Can you work these out from the model? Positions are in its coordinate system, mm. A direction names the side the tool comes from. Round coordinates to 2 decimals unless told otherwise and drop trailing zeros. Order: outer loops, then holes, each group sorted by start corner. A loop starts at its lowest first (then second) coordinate and runs counter-clockwise, first axis right, second up.
Q1. If we section it at C-C (z = 332): Please give me the cut outline in (x, y), plus the area to 3 significant figures.
Q2. We'd pull the mould along Z, two halves only. Please class faces 4 (the face through (-856, 0, -168)), 5 (the face through (-5, 6.35, 2)), 6 (the face through (819, 6.35, 2)), 7 (the face through (-17, 163, -190.5)): pulls with the +Z half, pulls with the -Z half, needs draft (parallel to the pull), parting line crosses it, or undercut.
Q3. If we section it at B-B (z = -5): Please give me the cut outline in (x, y), plus the area to 3 significant figures.
Q4. For faces 1 (the face through (-829, 6.35, 2)), 2 (the face through (-100.41, 240.65, 280.64)), 3 (the face through (-1233.488, 163, -3)), which set-ups out of +Z, -Z, +X, -X, +Y, -Y let a thin tool reach every point of the face, with its end or its side?
Q5. If I drill on line 1 (Y direction, x = -34, z = -142); line 2 (Z direction, x = -452.5, y = 53.5); line 3 (Y direction, x = -56.5, z = 498.5), over which ranges is the centre line in solid material (lowest first)?
Q6. Will these pins go through, and if not, where does the flat tip stop? P1, Ø12, axis at x = 708, y = 263.5, coming from the +Z side; P2, Ø8, axis at x = -379, z = -47.5, coming from the +Y side.
Q7. If we section it at A-A (x = 56.5): Please give me the cut outline in (y, z), plus the area to 3 significant figures.
from build123d import *

# Parameters (mm, degrees)
F0_W     = 2466.975
F0_H     = 381
F1_DEPTH = 330.2
F2_W     = 3.175
F2_H     = 381
F3_DEPTH = 12.7
F4_W     = 768.35
F4_H     = 330.2
F4_W_2   = 771.525
F5_DEPTH = 6.35
F6_R     = 76.2


with BuildPart() as f1:
    # F0 (on Front) → F1 (new body)
    with BuildSketch(Plane.XZ):
        Rectangle(F0_W, F0_H)
    extrude(amount=-F1_DEPTH)

    # F2 (on face) → F3 (cut)
    with BuildSketch(Plane.XZ):
        with Locations((-412.75, 0)):
            Rectangle(F2_W, F2_H)
        with Locations((412.75, 0)):
            Rectangle(F2_W, F2_H)
    extrude(amount=-F3_DEPTH, mode=Mode.SUBTRACT)

    # F4 (on face) → F5 (cut)
    with BuildSketch(Plane.XZ):
        with Locations((-823.9125, 0)):
            Rectangle(F4_W, F4_H)
        Rectangle(F4_W_2, F4_H)
        with Locations((823.9125, 0)):
            Rectangle(F4_W, F4_H)
    extrude(amount=-F5_DEPTH, mode=Mode.SUBTRACT)

    # F9: sweep along a path in F8
    with BuildLine(Plane(origin=(-90.4875, 0, 0), x_dir=(0, -1, 0), z_dir=(-1, 0, 0))) as f9_path:
        Line((-165.1, 190.5), (-165.1, 368.3))
        ThreePointArc((-165.1, 368.3), (-204.5570431921, 465.6007688069), (-300.6395792471, 507.9380352882))
        Line((-300.6395792471, 507.9380352882), (-330.2, 508.8187680178))
    # F6 (on face) → F9 (sweep)
    with BuildSketch(Plane.XY.offset(190.5)):
        with Locations((-90.4875, 165.1)):
            Circle(F6_R)
    sweep(path=f9_path.line)


solid = f1.part
Solution:
1. outline: circle Ø152.4 at (-90.49, 165.1)
1. area: 18,200 mm2
2. face 4: needs draft
2. face 5: undercut
2. face 6: undercut
2. face 7: pulls with the -Z half
3. outline: (-1233.49, 0) - (-1208.09, 0) - (-1208.09, 6.35) - (-439.74, 6.35) - (-439.74, 0) - (-414.34, 0) - (-414.34, 12.7) - (-411.16, 12.7) - (-411.16, 0) - (-385.76, 0) - (-385.76, 6.35) - (385.76, 6.35) - (385.76, 0) - (411.16, 0) - (411.16, 12.7) - (414.34, 12.7) - (414.34, 0) - (439.74, 0) - (439.74, 6.35) - (1208.09, 6.35) - (1208.09, 0) - (1233.49, 0) - (1233.49, 330.2) - (-1233.49, 330.2) - close
3. area: 800,000 mm2
4. face 1: -Y
4. face 2: none
4. face 3: +Z, -Z, -X, +Y, -Y
5. line 1: y = 6.35 to 330.2
5. line 2: z = -190.5 to 190.5
5. line 3: y = 142.72 to 330.51
6. P1: stops at z = 190.5
6. P2: stops at y = 330.2
7. outline: (0, -190.5) - (330.2, -190.5) - (330.2, 190.5) - (0, 190.5) - (0, 165.1) - (6.35, 165.1) - (6.35, -165.1) - (0, -165.1) - close
7. area: 124,000 mm2
